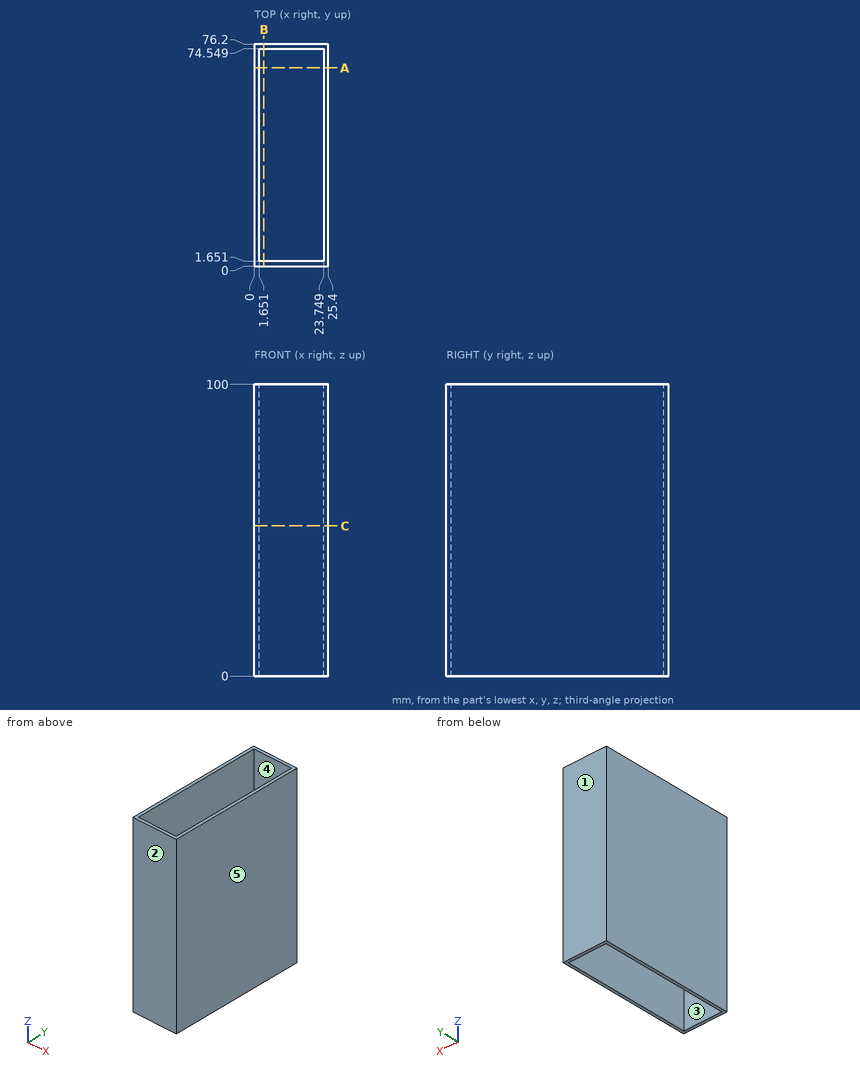
Job drawing, mm, ordinate dimensions from the low corner. One solid piece. A direction names the side the tool comes from. Give positions to 0.01 mm unless a question says otherwise; leave off trailing zeros. Order: outer loops, then holes, each group sorted by start corner. A loop starts at its lowest first (then second) coordinate and runs counter-clockwise, first axis right, second up. Notation, with made-up numbers: M 8.5,81.5 L 28.5,81.5 A17 ccw 28.5,93.5 Z; hole C -3.75,83 d11. An arc over 180 degrees is marked long. Put each result on its own line as item: value. Start each with the question number.
(1) Drill centre lines: L1, parallel to Y at x = 15.25, z = 24; L2, parallel to X at y = 14.5, z = 89. Where is each one in solid material? Low to high. Write a range as [from, to].
(2) Band-saw the part on C-C on z = 51.5. Give the cut face in (x, y).
(3) Tool access for the marked faces 4 and 5: list every direction of +Z, -Z, +X, -X, +Y, -Y with a clear straight run to the whole face (end or side of a thin tool).
(4) Band-saw the part on B-B on x = 3.25. Give the cut face in (y, z), then the cut area to 3 significant figures.
(5) Pull direction Y, two halves, no side cores. Call the marked faces 1, 2 and 3: released by +Y, released by -Y, zero draft, split by the parting line, or undercut.
(6) Band-saw the part on A-A on y = 68. Give the cut face in (x, z).
Results below:
1. L1: y = [0, 1.65], [74.55, 76.2]
1. L2: x = [0, 1.65], [23.75, 25.4]
2. outline: M 0,0 L 25.4,0 L 25.4,76.2 L 0,76.2 Z; hole M 1.65,1.65 L 23.75,1.65 L 23.75,74.55 L 1.65,74.55 Z
3. face 4: +Z, -Z
3. face 5: +Z, -Z, +X, +Y, -Y
4. outline: M 0,0 L 1.65,0 L 1.65,100 L 0,100 Z; M 74.55,0 L 76.2,0 L 76.2,100 L 74.55,100 Z
4. area: 330 mm2
5. face 1: released by +Y
5. face 2: released by -Y
5. face 3: undercut
6. outline: M 0,0 L 1.65,0 L 1.65,100 L 0,100 Z; M 23.75,0 L 25.4,0 L 25.4,100 L 23.75,100 Z
